Read the model definition and answer for the solid it produces. Units are mm, in the model's axes. Give positions to 0.01 mm unless a question says otherwise; leave off trailing zeros. Order: outer loops, then holes, each group sorted by start corner. A loop starts at its lowest first (then second) coordinate and runs counter-clockwise, first axis right, second up. Notation, with made-up numbers: M 20,40.25 L 38,40.25 A11 ccw 38,47.25 Z; hole C -20,35.5 d10. An arc over 180 degrees is marked long. One line per item, written item: value. Start each with the question number.
from build123d import *

# Parameters (mm, degrees)
BOSS_EXTRUDE1_DEPTH = 6
SKETCH2_W           = 6.2
SKETCH2_H           = 85
CUT_EXTRUDE1_DEPTH  = 6
SKETCH3_R           = 2
CUT_EXTRUDE2_DEPTH  = 6
SKETCH4_W           = 6
SKETCH4_H           = 136.9
SKETCH4_H_2         = 133.8
SKETCH4_H_3         = 137.464807664
BOSS_EXTRUDE2_DEPTH = 28
SKETCH5_W           = 6
SKETCH5_H           = 560
BOSS_EXTRUDE3_DEPTH = 28
SKETCH6_W           = 6
SKETCH6_H           = 0.564807664
CUT_EXTRUDE3_DEPTH  = 28
SKETCH7_W           = 6
SKETCH7_H           = 10
CUT_EXTRUDE4_DEPTH  = 1000


with BuildPart() as part:
    # Sketch1 → Boss-Extrude1 (new body)
    with BuildSketch(Plane(origin=(0, 0, 0), x_dir=(0, 0, -1), z_dir=(1, 0, 0))):
        Polygon((0, 0), (560, 0), (560, 10), (578, 10), (578, 85), (571.9, 85), (571.9, 160), (560, 160), (560, 170), (0, 170), (0, 160), (-11.9, 160), (-11.9, 85), (-18, 85), (-18, 10), (0, 10), align=None)
    extrude(amount=BOSS_EXTRUDE1_DEPTH)

    # Sketch2 → Cut-Extrude1 (cut)
    with BuildSketch(Plane(origin=(6, 0, 0), x_dir=(0, 0, -1), z_dir=(1, 0, 0))):
        with Locations((140, 127.5)):
            Rectangle(SKETCH2_W, SKETCH2_H)
        with Locations((280, 127.5)):
            Rectangle(SKETCH2_W, SKETCH2_H)
        with Locations((420, 127.5)):
            Rectangle(SKETCH2_W, SKETCH2_H)
    extrude(amount=-CUT_EXTRUDE1_DEPTH, mode=Mode.SUBTRACT)

    # Sketch3 → Cut-Extrude2 (cut)
    with BuildSketch(Plane(origin=(6, 0, 0), x_dir=(0, 0, -1), z_dir=(1, 0, 0))):
        with Locations((68.45, 130)):
            Circle(SKETCH3_R)
        with Locations((68.45, 40)):
            Circle(SKETCH3_R)
        with Locations((210, 130)):
            Circle(SKETCH3_R)
        with Locations((210, 40)):
            Circle(SKETCH3_R)
        with Locations((350, 130)):
            Circle(SKETCH3_R)
        with Locations((350, 40)):
            Circle(SKETCH3_R)
        with Locations((491.55, 130)):
            Circle(SKETCH3_R)
        with Locations((491.55, 40)):
            Circle(SKETCH3_R)
    extrude(amount=-CUT_EXTRUDE2_DEPTH, mode=Mode.SUBTRACT)

    # Sketch4 → Boss-Extrude2 (add)
    with BuildSketch(Plane(origin=(0, 170, 0), x_dir=(1, 0, 0), z_dir=(0, 1, 0))):
        with Locations((3, 68.45)):
            Rectangle(SKETCH4_W, SKETCH4_H)
        with Locations((3, 210)):
            Rectangle(SKETCH4_W, SKETCH4_H_2)
        with Locations((3, 350)):
            Rectangle(SKETCH4_W, SKETCH4_H_2)
        with Locations((3, 491.267596168)):
            Rectangle(SKETCH4_W, SKETCH4_H_3)
    extrude(amount=BOSS_EXTRUDE2_DEPTH)

    # Sketch5 → Boss-Extrude3 (add)
    with BuildSketch(Plane.XZ):
        with Locations((3, -280)):
            Rectangle(SKETCH5_W, SKETCH5_H)
    extrude(amount=BOSS_EXTRUDE3_DEPTH)

    # Sketch6 → Cut-Extrude3 (cut)
    with BuildSketch(Plane.XZ.offset(-170)):
        with Locations((3, -422.817596168)):
            Rectangle(SKETCH6_W, SKETCH6_H)
    extrude(amount=-CUT_EXTRUDE3_DEPTH, mode=Mode.SUBTRACT)

    # Sketch7 → Cut-Extrude4 (cut)
    with BuildSketch(Plane(origin=(0, 0, -560), x_dir=(-1, 0, 0), z_dir=(0, 0, -1))):
        with Locations((-3, 193)):
            Rectangle(SKETCH7_W, SKETCH7_H)
        with Locations((-3, -23)):
            Rectangle(SKETCH7_W, SKETCH7_H)
    extrude(amount=-CUT_EXTRUDE4_DEPTH, mode=Mode.SUBTRACT)


solid = part.part
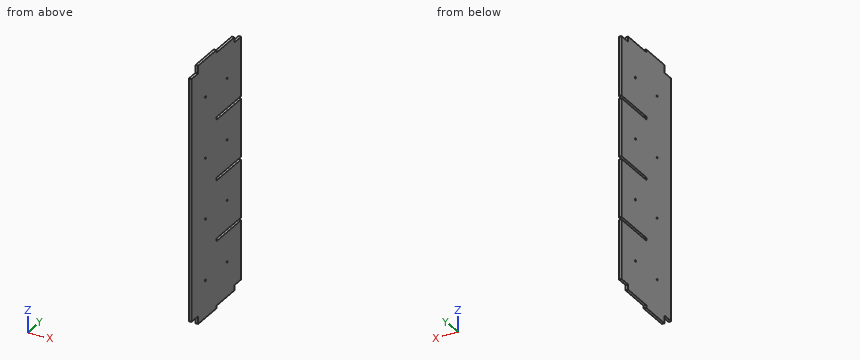
Q1. Find section A-A, the plane y = 91. Give the vertices of the cut face in (x, z), then the cut area to 3 significant figures.
Q2. Consider probe 1 along Y at (x, z) = (0.6, -492); probe 2 along Z at (x, y) = (0.45, 144); probe 3 along Y at (x, z) = (2.7, -68.45). Determine where each line is inside the solid, lowest interval first.
Q3. Each of these flat-tipped pins is pushed along its axis until it touches: pin 1 (3 mm diameter, centred on x = 2, y = 172, fed in from +Z); pin 2 (1.8 mm diameter, centred on x = 2, z = -569, fed in from -Y); pin 3 (1.5 mm diameter, centred on y = 150, z = -375.5, fed in from -X); pin 4 (2 mm diameter, centred on x = 3, y = 133.5, fed in from -Z). Where does it stop, or does it pass through?
Q4. Find section B-B, the plane x = 2.35. State how many separate pieces and enclosed holes the cut face has, then the cut area to 3 significant figures.
Evaluation:
1. outline: M 0,-571.9 L 6,-571.9 L 6,-423.1 L 0,-423.1 Z; M 0,-416.9 L 6,-416.9 L 6,-283.1 L 0,-283.1 Z; M 0,-276.9 L 6,-276.9 L 6,-143.1 L 0,-143.1 Z; M 0,-136.9 L 6,-136.9 L 6,11.9 L 0,11.9 Z
1. area: 3,390 mm2
2. probe 1: -18 to 38.05, 41.95 to 128.05, 131.95 to 188
2. probe 2: -571.9 to -423.1, -416.9 to -283.1, -276.9 to -143.1, -136.9 to 11.9
2. probe 3: -18 to 38, 42 to 128, 132 to 188
3. pin 1: z = 0
3. pin 2: y = 10
3. pin 3: x = 0
3. pin 4: z = -571.9
4. separate pieces: 1
4. enclosed holes: 8
4. area: 118,000 mm2
